The listing builds one solid part. Answer for the finished solid, in the listing's coordinates (mm). A direction names the side the tool comes from. Coordinates: 2 decimals unless noted, no trailing zeros. Write each loop counter-clockwise with the first axis right and the second up, starting at its lowest first coordinate (ties: lowest second). Pieces come first, ordered by that corner, then holes.
Autodesk Inventor part; units mm, degrees
ref_plane "YZ Plane" through (0, 0, 0) normal (1, 0, 0) x (0, 1, 0)
ref_plane "XZ Plane" through (0, 0, 0) normal (0, 1, 0) x (-1, 0, 0)
ref_plane "XY Plane" through (0, 0, 0) normal (0, 0, 1) x (1, 0, 0)
sketch "Sketch_1" plane through (0, 0, 0) normal (0, 0, 1) x (1, 0, 0)
  line L0 (234, 0) -> (0, 0)
  line L1 (0, 0) -> (0, 4.5)
  line L2 (0, 4.5) -> (0.5, 5)
  line L3 (0.5, 5) -> (233.5, 5)
  line L4 (233.5, 5) -> (234, 4.5)
  line L5 (234, 4.5) -> (234, 0)
  line L6 (234, 0) -> (0, 0)
revolve "Revolution1" add sketch "Sketch_1" angle 360 about axis through (234, 0, 0) along (1, 0, 0)
sketch "Sketch2" plane through (0, 0, 0) normal (-1, 0, 0) x (0, 0, 1)
  point P0 (0, 0)
hole "Hole1" at (0, 0, 0) direction (1, 0, 0) diameter 4.917 depth 17.5806 tip angle 120 countersink diameter 6 countersink angle 90
sketch "Sketch3" plane through (234, 0, 0) normal (1, 0, 0) x (0, 0, -1)
  point P0 (0, 0)
hole "Hole2" at (234, 0, 0) direction (-1, 0, 0) diameter 4.917 depth 23.5806 tip angle 120 countersink diameter 6 countersink angle 90
properties part number "SSFMRW10-234-M6-ND6_s"
Q1. Which of the six approach directions +Z, -Z, +X, -X, +Y, -Y give full straight-line access (tool end or side, diameter ignored) to faces 1 (the face through (9.18, -0.738, 2.345)), 2 (the face through (234, 1, -3)), 3 (the face through (221.778, -0.738, -2.345))?
Answers below:
face 1: -X
face 2: +Z, -Z, +X, +Y, -Y
face 3: +X
Q2. The part is cut by section A-A, the plane x = 147.5. Write down the section's boundary in (y, z).
Answers below:
outline: circle Ø10 at (0, 0)
Q3. Find the intervals of material crossed by probe 1 along Z at (x, y) = (11, 0); probe 2 along Z at (x, y) = (104, -0.25); probe 3 along Z at (x, y) = (71, 4), in increasing order.
Answers below:
probe 1: z = -5 to -2.46, 2.46 to 5
probe 2: z = -4.99 to 4.99
probe 3: z = -3 to 3
Q4. Given pin 1 (1.5 mm diameter, centred on x = 38.5, y = 3, fed in from +Z); pin 2 (4.5 mm diameter, centred on y = 0, z = 0, fed in from +X); pin 3 (1 mm diameter, centred on x = 39, z = 2.5, fed in from -Y), each flat-ended and moving along its own axis, determine where each tip first touches the part or whether it passes through.
Answers below:
pin 1: stops at z = 4.47
pin 2: stops at x = 210.3
pin 3: stops at y = -4.58
Q5. Determine the mould class of faces 4 (the face through (0, 1, -3)), 5 (the face through (209, 0, 0)), 6 (the face through (118.63, -1.08, -4.88)) for opening direction Z: released by +Z, released by -Z, zero draft, split by the parting line, or undercut.
Answers below:
face 4: zero draft
face 5: undercut
face 6: split by the parting line
